Autodesk Inventor part; units mm, degrees
ref_plane "YZ Plane" through (0, 0, 0) normal (1, 0, 0) x (0, 1, 0)
ref_plane "XZ Plane" through (0, 0, 0) normal (0, 1, 0) x (-1, 0, 0)
ref_plane "XY Plane" through (0, 0, 0) normal (0, 0, 1) x (1, 0, 0)
sketch "Sketch1" plane through (0, 0, 0) normal (0, 0, 1) x (1, 0, 0)
  circle A0 centre (0, 0) radius 44.45
  dimension "d0" = 88.9
extrude "Extrusion1" add sketch "Sketch1" along normal blind 19.05
sketch "Sketch2" plane through (0, 0, 19.05) normal (0, 0, 1) x (1, 0, 0)
  circle A0 centre (0, 34.29) radius 3.4925
  circle A1 centre (0, -34.29) radius 3.4925
  point P0 (0, 0)
  dimension "d3" = 6.985
  dimension "d4" = 34.29
  dimension "d5" = 6.985
  dimension "d6" = 34.29
sketch "Sketch3" plane through (0, 0, 19.05) normal (0, 0, 1) x (1, 0, 0)
  circle A0 centre (0, 0) radius 44.45
  dimension "d9" = 88.9
extrude "Extrusion3" cut sketch "Sketch3" against normal blind 8.89
sketch "Sketch4" plane through (0, 0, 10.16) normal (0, 0, 1) x (1, 0, 0)
  circle A0 centre (0, 0) radius 6.35
  dimension "d12" = 12.7
extrude "Extrusion4" cut sketch "Sketch2" against normal blind 26.9875
extrude "Extrusion5" cut sketch "Sketch4" against normal blind 44.45
sketch "Sketch5" plane through (0, 0, 10.16) normal (0, 0, 1) x (1, 0, 0)
  circle A0 centre (-30.48, 0) radius 4.445
  circle A1 centre (0, 0) radius 6.35
  circle A2 centre (0, 34.29) radius 3.4925
  line L0 (0, 0) -> (0, 34.29)
  circle A3 centre (30.48, 0) radius 4.445
  dimension "d17" = 8.89
  dimension "d18" = 30.48
  dimension "d19" = 34.29
extrude "Extrusion6" cut sketch "Sketch5" against normal blind 80.9625 contours A0 | A3
sketch "Sketch6" plane through (0, 0, 10.16) normal (0, 0, 1) x (1, 0, 0)
  circle A0 centre (-30.48, 0) radius 8.89
  circle A1 centre (0, 34.29) radius 3.4925
  line L0 (0, 0) -> (0, 34.29)
  circle A2 centre (30.48, 0) radius 8.89
  circle A3 centre (-30.48, 0) radius 4.445
  circle A4 centre (-30.48, 0) radius 4.445
  circle A5 centre (30.48, 0) radius 4.445
  dimension "d22" = 17.78
  dimension "d23" = 30.48
  dimension "d24" = 34.29
  dimension "d25" = 0
extrude "Extrusion7" cut sketch "Sketch6" against normal blind 6.35 contours A0 | A2
sketch "Sketch8" plane through (-30.48, 0, 3.81) normal (0, 0, 1) x (1, 0, 0)
  circle A0 centre (0, 0) radius 4.445
  circle A1 centre (0, 0) radius 8.89
  circle A2 centre (0, 0) radius 4.445
  circle A3 centre (0, 0) radius 8.89
  circle A4 centre (30.48, 34.29) radius 3.4925
  line L0 (30.48, 34.29) -> (30.48, 0)
  circle A5 centre (60.96, 0) radius 4.445
  circle A6 centre (60.96, 0) radius 8.89
  dimension "d28" = 0
  dimension "d29" = 0
  dimension "d30" = 30.48
  dimension "d31" = 34.29
extrude "Extrusion8" add sketch "Sketch8" against normal blind 7.62 contours A1 | A6
properties part number "Crank"
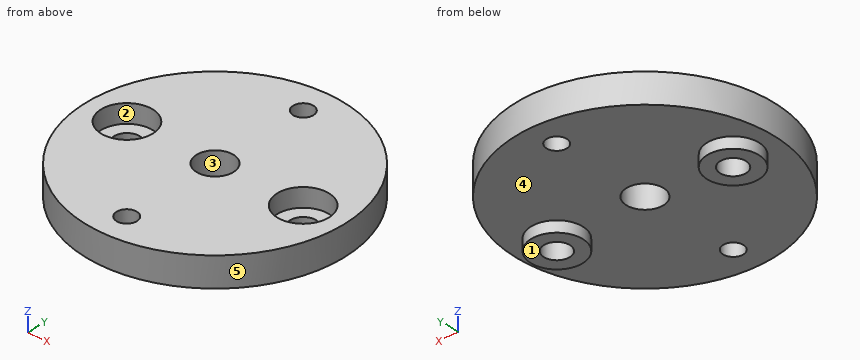
Part model, mm, in its own coordinate system. Face numbers are marked on the shaded views. A direction names the side the tool comes from. Give positions to 0.01 mm unless a question says otherwise; leave off trailing zeros. Order: outer loops, then holes, each group sorted by start corner. A loop starts at its lowest first (then second) coordinate and runs counter-clockwise, first axis right, second up. Notation, with made-up numbers: (71.25, 79.25) - (117.25, 79.25) arc R12 ccw to (117.25, 86.25) - close; hole circle Ø9 at (39, 21). An arc over 180 degrees is marked (long way). Use one line per item in the form item = value.
Item 1: Pin check, flat tips, straight feed: pin 1 Ø8 at (x, y) = (0, 34.29) entering from -Z; pin 2 Ø11.5 at (x, y) = (-30.48, 0) entering from +Z; pin 3 Ø2 at (x, z) = (-16, 0.5) entering from +Y; pin 4 Ø9 at (x, y) = (0, -34.29) entering from +Z. Stop position of each tip, or through.
Solution:
pin_1 = 0
pin_2 = 3.81
pin_3 = 41.84
pin_4 = 10.16
Item 2: Probe probe 1 along Y at (x, z) = (0, 5.5); probe 2 along Y at (x, z) = (30.48, -1.5) (3 decimals); probe 3 along Y at (x, z) = (1, 9.25). List the from-to ranges inside material, lowest first. Write a range as from..to.
Solution:
probe_1 = -44.45..-37.78, -30.8..-6.35, 6.35..30.8, 37.78..44.45
probe_2 = -8.89..-4.445, 4.445..8.89
probe_3 = -44.44..-37.64, -30.94..-6.27, 6.27..30.94, 37.64..44.44
Item 3: Slice it at D-D on y = -34.29. Give the cut face in (x, z), and give its area (3 significant figures).
Solution:
outline = (-28.28, 0) - (-3.49, 0) - (-3.49, 10.16) - (-28.28, 10.16) - close; (3.49, 0) - (28.28, 0) - (28.28, 10.16) - (3.49, 10.16) - close
area = 504 mm2
Item 4: Two-plate mould, pull along Y, no slides. Class the marked faces 3, 4 and 5: released by +Y, released by -Y, zero draft, split by the parting line, or undercut.
Solution:
face_3 = undercut
face_4 = zero draft
face_5 = split by the parting line
Item 5: Slice it at A-A on x = 0. Give the cut face in (y, z).
Solution:
outline = (-44.45, 0) - (-37.78, 0) - (-37.78, 10.16) - (-44.45, 10.16) - close; (-30.8, 0) - (-6.35, 0) - (-6.35, 10.16) - (-30.8, 10.16) - close; (6.35, 0) - (30.8, 0) - (30.8, 10.16) - (6.35, 10.16) - close; (37.78, 0) - (44.45, 0) - (44.45, 10.16) - (37.78, 10.16) - close
Item 6: Slice it at B-B on y = 0. Count the separate pieces of the cut face and the enclosed holes in it, and give its area (3 significant figures).
Solution:
separate_pieces = 4
enclosed_holes = 0
area = 548 mm2
Item 7: Which spindle directions (+Z, -Z, +X, -X, +Y, -Y) get a long thin tool onto all of the face, cutting with end or side? Do the marked faces 1 and 2. Say none if no direction does.
Solution:
face_1 = -Z, +X, -X, +Y, -Y
face_2 = +Z
